For this review, take the finished solid that the model builds, in its own axes (mm). A direction names the side the tool comes from. Give positions to 0.01 mm unless a question says otherwise; leave off trailing zeros. Loops run counter-clockwise (first coordinate to the right, second up) from the corner with the lowest first, then second, coordinate; pieces in that order, holes last.
```python
from build123d import *

# Parameters (mm, degrees)
SKETCH4_R           = 21.5
SKETCH4_R_2         = 1.45
BOSS_EXTRUDE1_DEPTH = 4
BOSS_EXTRUDE2_DEPTH = 4
CUT_EXTRUDE1_DEPTH  = 1.5


with BuildPart() as part:
    # Sketch4 → Boss-Extrude1 (new body)
    with BuildSketch(Plane.XY):
        Circle(SKETCH4_R)
        with Locations((-12.727922061, 12.727922061)):
            Circle(SKETCH4_R_2, mode=Mode.SUBTRACT)
        with BuildLine():
            Line((-1.6, -2.1), (-1.6, 2.1))
            ThreePointArc((-1.6, 2.1), (0, 2.625143683), (1.6, 2.1))
            Line((1.6, 2.1), (1.6, -2.1))
            ThreePointArc((1.6, -2.1), (0, -2.625143683), (-1.6, -2.1))
        make_face(mode=Mode.SUBTRACT)
    extrude(amount=BOSS_EXTRUDE1_DEPTH)

    # Sketch5 → Boss-Extrude2 (add)
    with BuildSketch(Plane.XY.offset(4)):
        with BuildLine():
            ThreePointArc((-14.24122807, -0.499923047), (10.076271632, -10.076271632), (0.499923047, 14.24122807))
            ThreePointArc((0.499923047, 14.24122807), (-3.820227547, 3.820227547), (-14.24122807, -0.499923047))
        make_face()
        with BuildLine():
            Line((1.6, -2.1), (1.6, 2.1))
            ThreePointArc((1.6, 2.1), (0, 2.625143683), (-1.6, 2.1))
            Line((-1.6, 2.1), (-1.6, -2.1))
            ThreePointArc((-1.6, -2.1), (0, -2.625143683), (1.6, -2.1))
        make_face(mode=Mode.SUBTRACT)
    extrude(amount=BOSS_EXTRUDE2_DEPTH)

    # Sketch7 → Cut-Extrude1 (cut)
    with BuildSketch(Plane(origin=(0, 0, 0), x_dir=(-1, 0, 0), z_dir=(0, 0, -1))):
        with BuildLine():
            Line((-1.6, -2.081196616), (-1.6, 2.081196616))
            ThreePointArc((-1.6, 2.081196616), (-2.625143683, 0), (-1.6, -2.081196616))
        make_face()
        with BuildLine():
            ThreePointArc((2.625143683, 0), (2.354953211, 1.159989108), (1.6, 2.081196616))
            Line((1.6, 2.081196616), (1.6, -2.081196616))
            ThreePointArc((1.6, -2.081196616), (2.354953211, -1.159989108), (2.625143683, 0))
        make_face()
    extrude(amount=-CUT_EXTRUDE1_DEPTH, mode=Mode.SUBTRACT)


solid = part.part
```
Item 1: Take a section at A-A on x = 0. Give the boundary of the cut face in (y, z).
Answer:
outline: (-21.5, 0) - (-2.63, 0) - (-2.63, 8) - (-14.25, 8) - (-14.25, 4) - (-21.5, 4) - close; (2.63, 0) - (21.5, 0) - (21.5, 4) - (10.44, 4) - (10.44, 8) - (2.63, 8) - close
Item 2: For L1, parallel to Z at x = 14, y = -5; L2, parallel to Y at x = 0, z = 1.5; L3, parallel to Y at x = 2, z = 1, list the stretches that pass through material, from the lowest coordinate up.
Answer:
L1: z = 0 to 4
L2: y = -21.5 to -2.63, 2.63 to 21.5
L3: y = -21.41 to -1.7, 1.7 to 21.41
Item 3: Clearance check with flat-ended pins moving along their axes: pin 1 Ø3 at (x, z) = (-2, 6) entering from -Y; pin 2 Ø3 at (x, z) = (-10, 1.5) entering from +Y; pin 3 Ø3 at (x, z) = (-8, 1) entering from +Y. State where each tip first meets the part, or that it passes through.
Answer:
pin 1: stops at y = -14.24
pin 2: stops at y = 19.75
pin 3: stops at y = 20.49
Item 4: The part is to be moulded in two halves that separate along X. For faces 5 (the flat face through (3, -3, 8)), 6 (the cylindrical face through (-3.706, 3.935, 5.972)), 7 (the flat face through (-2, 0, 1.5)), say which applies: released by +X, released by -X, zero draft, split by the parting line, or undercut.
Answer:
face 5: zero draft
face 6: released by -X
face 7: undercut
Item 5: Take a section at C-C on y = 6.5. Give the boundary of the cut face in (x, z).
Answer:
outline: (-20.49, 0) - (20.49, 0) - (20.49, 4) - (12.68, 4) - (12.68, 8) - (-1.7, 8) - (-1.7, 4) - (-20.49, 4) - close
Item 6: Tool access review of faces 1 (the flat face through (-5, 5, 4)), 2 (the cylindrical face through (2.625, 0.034, 0.74)), 3 (the cylindrical face through (0.024, 2.625, 3.944)), 4 (the flat face through (4, 0, 0)): name each direction out of +Z, -Z, +X, -X, +Y, -Y from which nothing blocks a thin tool from reaching the whole face with its end or side.
Answer:
face 1: +Z
face 2: -Z
face 3: +Z, -Z
face 4: -Z, +X, -X, +Y, -Y
Item 7: Take a section at B-B on z = 6. Give the boundary of the cut face in (x, y), and give its area (3 significant figures).
Answer:
outline: (-14.24, -0.5) arc R14.25 ccw (long way) to (0.5, 14.24) arc R14.75 cw to start; hole (-1.6, -2.1) arc R2.7 ccw to (1.6, -2.1) - (1.6, 2.1) arc R2.7 ccw to (-1.6, 2.1) - close
area: 495 mm2
Item 8: Take a section at D-D on y = -1.5. Give the boundary of the cut face in (x, z).
Answer:
outline: (-21.45, 0) - (-2.15, 0) - (-2.15, 1.5) - (-1.6, 1.5) - (-1.6, 8) - (-14.17, 8) - (-14.17, 4) - (-21.45, 4) - close; (1.6, 1.5) - (2.15, 1.5) - (2.15, 0) - (21.45, 0) - (21.45, 4) - (14.17, 4) - (14.17, 8) - (1.6, 8) - close
